```python
from build123d import *

# Parameters (mm, degrees)
SKETCH3_W                    = 914.4
SKETCH3_H                    = 609.6
BOSS_EXTRUDE1_DEPTH          = 0.79375
SKETCH4_OUTSIDE_W            = 1136.194
SKETCH4_OUTSIDE_H            = 831.394
CUT_EXTRUDE1_DEPTH           = 2.54
CUT_EXTRUDE2_DEPTH           = 2.54
CUT_EXTRUDE3_DEPTH           = 2.54
F_10_0_1935_DIAMETER_HOLE1_D = 4.9149
F_1_4_0_25_DIAMETER_HOLE1_D  = 6.35
F_10_CLEARANCE_HOLE1_D       = 4.9784


with BuildPart() as part:
    # Sketch3 → Boss-Extrude1 (new, symmetric)
    with BuildSketch(Plane.XY):
        Rectangle(SKETCH3_W, SKETCH3_H)
    extrude(amount=BOSS_EXTRUDE1_DEPTH, both=True)

    # Sketch4 outside → Cut-Extrude1 (cut)
    with BuildSketch(Plane.XY.offset(0.79375)):
        Rectangle(SKETCH4_OUTSIDE_W, SKETCH4_OUTSIDE_H)
        with BuildLine():
            Line((-326.734938229, -279.58151343), (-352.134938229, -254.18151343))
            Line((-352.134938229, -254.18151343), (-352.134938229, -29.709012922))
            ThreePointArc((-352.134938229, -29.709012922), (-351.390989453, -27.912961698), (-349.594938229, -27.169012922))
            Line((-349.594938229, -27.169012922), (331.125061771, -27.169012922))
            ThreePointArc((331.125061771, -27.169012922), (332.921112995, -27.912961698), (333.665061771, -29.709012922))
            Line((333.665061771, -29.709012922), (333.665061771, -254.18151343))
            Line((333.665061771, -254.18151343), (308.265061771, -279.58151343))
            Line((308.265061771, -279.58151343), (-326.734938229, -279.58151343))
        make_face(mode=Mode.SUBTRACT)
    extrude(amount=-CUT_EXTRUDE1_DEPTH, mode=Mode.SUBTRACT)

    # Sketch7 → Cut-Extrude2 (cut)
    with BuildSketch(Plane.XY.offset(0.79375)):
        with BuildLine():
            Line((-269.584938229, -195.44401343), (-374.359938229, -195.44401343))
            Line((-374.359938229, -195.44401343), (-374.359938229, -4.94401343))
            Line((-374.359938229, -4.94401343), (-183.859938229, -4.94401343))
            Line((-183.859938229, -4.94401343), (-183.859938229, -109.71901343))
            ThreePointArc((-183.859938229, -109.71901343), (-208.968209412, -170.335742247), (-269.584938229, -195.44401343))
        make_face()
    extrude(amount=-CUT_EXTRUDE2_DEPTH, mode=Mode.SUBTRACT)

    # Sketch8 → Cut-Extrude3 (cut)
    with BuildSketch(Plane.XY.offset(0.79375)):
        with BuildLine():
            Line((251.115061771, -195.44401343), (355.890061771, -195.44401343))
            Line((355.890061771, -195.44401343), (355.890061771, -4.94401343))
            Line((355.890061771, -4.94401343), (165.390061771, -4.94401343))
            Line((165.390061771, -4.94401343), (165.390061771, -109.71901343))
            ThreePointArc((165.390061771, -109.71901343), (190.498332954, -170.335742247), (251.115061771, -195.44401343))
        make_face()
    extrude(amount=-CUT_EXTRUDE3_DEPTH, mode=Mode.SUBTRACT)

    # #10 (0.1935) Diameter Hole1 (through all)
    with Locations(Plane.XY.offset(0.79375)):
        with Locations((-288.634938229, -266.88151343), (-314.034938229, -266.88151343), (-339.434938229, -254.18151343), (89.952061771, -268.113109138), (115.352061771, -268.113109138), (218.222061771, -266.881513934), (243.622061771, -266.881513934), (295.565061771, -266.88151343), (270.165061771, -266.88151343), (320.965061771, -254.18151343), (124.115061771, -39.86901343), (-142.584938737, -39.86901343), (-60.034938737, -266.88151343), (41.565061263, -266.88151343)):
            Hole(F_10_0_1935_DIAMETER_HOLE1_D / 2)

    # 1/4 (0.25) Diameter Hole1 (through all)
    with Locations(Plane.XY.offset(0.79375)):
        with Locations((-339.434938229, -204.969013938), (320.965061771, -204.96901343), (155.865061771, -39.86901343), (-174.334938229, -39.86901343)):
            Hole(F_1_4_0_25_DIAMETER_HOLE1_D / 2)

    # #10 Clearance Hole1 (through all)
    with Locations(Plane.XY.offset(0.79375)):
        with Locations((-117.184938229, -204.17526343), (-117.184938229, -102.57526343), (98.715061771, -102.57526343), (98.715061771, -204.17526343), (230.160061773, -238.782763436), (287.31006177, -210.842763429)):
            Hole(F_10_CLEARANCE_HOLE1_D / 2)


solid = part.part
```
CAD build for the part. Positions are in the model's coordinates, mm. Coordinates: 2 decimals unless noted, no trailing zeros. Write each loop counter-clockwise with the first axis right and the second up, starting at its lowest first coordinate (ties: lowest second). Pieces come first, ordered by that corner, then holes. Notation, with made-up numbers: (-11.5, -20) -> (7.5, -20) arc R20 cw to (7.5, -1) -> close; hole circle Ø10 at (82.25, 3). An arc over 180 degrees is marked (long way). Use CSV: the item, a comma, the result in double quotes. Start each with the question number.
Item 1: Band-saw the part on C-C, the plane y = -143. Write the cut outline in (x, z), plus the area to 3 significant figures.
Item 2: Wall check: probe 1 along X at (y, z) = (-103, -0.2); probe 2 along X at (y, z) = (-252, -0.45); probe 3 along Y at (x, z) = (116, 0.7). Give the ranges that are in metal, low to high.
Item 3: Drop flat-ended pins along their axis: P1, Ø10, axis at x = -188, y = -103.5, coming from the -Z side; P2, Ø0.8, axis at x = -331, z = 0, coming from the +Y side. Give the stop position or say it passes through.
Item 4: Band-saw the part on A-A, the plane y = -176.5. Write the cut outline in (x, z).
Item 5: Band-saw the part on B-B, the plane z = -0.5. Give the number of separate pieces and of enclosed holes in the cut face, plus the area to 3 significant figures.
Response values:
1,outline,"(-190.58, -0.79) -> (172.11, -0.79) -> (172.11, 0.79) -> (-190.58, 0.79) -> close"
1,area,"576 mm2"
2,probe 1,"x = -183.86 to -119.64, -114.73 to 96.26, 101.17 to 165.39"
2,probe 2,"x = -352.13 to -340.57, -338.3 to 319.83, 322.1 to 333.67"
2,probe 3,"y = -279.58 to -270.48, -265.74 to -27.17"
3,P1,"stops at z = -0.79"
3,P2,"stops at y = -195.44"
4,outline,"(-215.83, -0.79) -> (197.36, -0.79) -> (197.36, 0.79) -> (-215.83, 0.79) -> close"
5,separate pieces,"1"
5,enclosed holes,"24"
5,area,"118,000 mm2"
